Read the model definition and answer for the solid it produces. Units are mm, in the model's axes. A direction names the side the tool comes from. Give positions to 0.01 mm unless a question says otherwise; leave off trailing zeros. Loops run counter-clockwise (first coordinate to the right, second up) from the corner with the lowest first, then second, coordinate; pieces in that order, holes last. Notation, with made-up numbers: M -18.5,-31.5 L 38.5,-31.5 A34 ccw 38.5,5.5 Z; hole C -32,85 d7. An arc over 180 degrees is marked long. Return JSON: item names as keys, results as strings. Group by question number.
```python
from build123d import *

# Parameters (mm, degrees)
F3_DEPTH = 2.5
F4_DEPTH = 5


with BuildPart() as f1:
    # F0 (on Front) → F1 (revolve)
    with BuildSketch(Plane.XZ):
        with BuildLine():
            Line((8.5, 0), (5, 0))
            Line((5, 0), (5, -3.5))
            Line((5, -3.5), (12, -3.5))
            ThreePointArc((12, -3.5), (9.5251262658, -2.4748737342), (8.5, 0))
        make_face()
    revolve(axis=Axis((0, 0, 10.7058882713), (0, 0, 1)))

    # F2 (on face) → F3 (cut)
    with BuildSketch(Plane.XY):
        with BuildLine():
            ThreePointArc((1, 7), (-0.0357371137, 7.9993612253), (-0.9974457174, 6.9285714286))
            ThreePointArc((-0.9974457174, 6.9285714286), (0, 6), (0.9974457174, 6.9285714286))
            ThreePointArc((0.9974457174, 6.9285714286), (0.9993612253, 6.9642628863), (1, 7))
        make_face()
        with BuildLine():
            ThreePointArc((-6, 0), (-6.2680749453, 0.6813851439), (-6.9285714286, 0.9974457174))
            ThreePointArc((-6.9285714286, 0.9974457174), (-8, 0), (-6.9285714286, -0.9974457174))
            ThreePointArc((-6.9285714286, -0.9974457174), (-6.2680749453, -0.6813851439), (-6, 0))
        make_face()
        with BuildLine():
            ThreePointArc((0.9974457174, -6.9285714286), (0, -6), (-0.9974457174, -6.9285714286))
            ThreePointArc((-0.9974457174, -6.9285714286), (-0.0357371137, -7.9993612253), (1, -7))
            ThreePointArc((1, -7), (0.9993612253, -6.9642628863), (0.9974457174, -6.9285714286))
        make_face()
        with BuildLine():
            ThreePointArc((8, 0), (7.6813851439, 0.7319250547), (6.9285714286, 0.9974457174))
            ThreePointArc((6.9285714286, 0.9974457174), (6, 0), (6.9285714286, -0.9974457174))
            ThreePointArc((6.9285714286, -0.9974457174), (7.6813851439, -0.7319250547), (8, 0))
        make_face()
    extrude(amount=-F3_DEPTH, mode=Mode.SUBTRACT)

    # F4 (add): faces of the model
    f4_faces = [f1.faces().sort_by_distance(p)[0] for p in [
        (0, 7, -2.5),
        (0, -7, -2.5),
    ]]
    extrude(f4_faces, amount=F4_DEPTH)


solid = f1.part
```
1. The mould has two halves that part along Y. Classify faces 3 (the flat face through (7, 0, -2.5)), 4 (the flat face through (0, 7, 2.5)): +Y half, -Y half, draft (parallel to the pull), parting line (faces both ways), or undercut.
2. For faces 1 (the flat face through (-5.2, 0.2, -3.5)), 2 (the flat face through (-7, 0, -2.5)), determine the directions among +Z, -Z, +X, -X, +Y, -Y from which every point of the face is accessible in a straight line to the end or side of a thin tool.
3. Flat-ended cylindrical pins translate along their axes: P1, Ø2, axis at x = 7.5, y = 0, coming from the +Z side; P2, Ø4, axis at x = 0, y = -2, coming from the +Z side. Find the tip coordinate at first contact, or state that the pin passes through.
4. Find section A-A (x = 0). Write down the section's boundary in (y, z), and give its area (3 significant figures).
5. Straight lines are drawn through the part: line 1 along X through (y, z) = (-3, -0.25); line 2 along Z through (x, y) = (7.5, -2); line 3 along Y through (x, z) = (0, -2.65). For each, find the intervals that lie inside material, in ascending order.
6. Find section B-B (z = -1). Write down the section's boundary in (x, y), and give its area (3 significant figures).
Result:
{
 "1": {"face 3": "undercut", "face 4": "draft"},
 "2": {"face 1": "-Z, +X, -X, +Y, -Y", "face 2": "+Z"},
 "3": {"P1": "stops at z = 0", "P2": "passes through"},
 "4": {"outline": "M -12,-3.5 L -5,-3.5 L -5,0 L -6,0 L -6,2.5 L -8,2.5 L -8,0 L -8.5,0 A3.5 cw Z; M 5,-3.5 L 12,-3.5 A3.5 cw 8.5,0 L 8,0 L 8,2.5 L 6,2.5 L 6,0 L 5,0 Z", "area": "39.8 mm2"},
 "5": {"line 1": "x = -7.96 to -4, 4 to 7.96", "line 2": "z = -3.5 to 0", "line 3": "y = -9.71 to -5, 5 to 9.71"},
 "6": {"outline": "C 0,0 d17.29; hole C -7,0 d2; hole C 0,0 d10; hole C 7,0 d2", "area": "150 mm2"}
}
